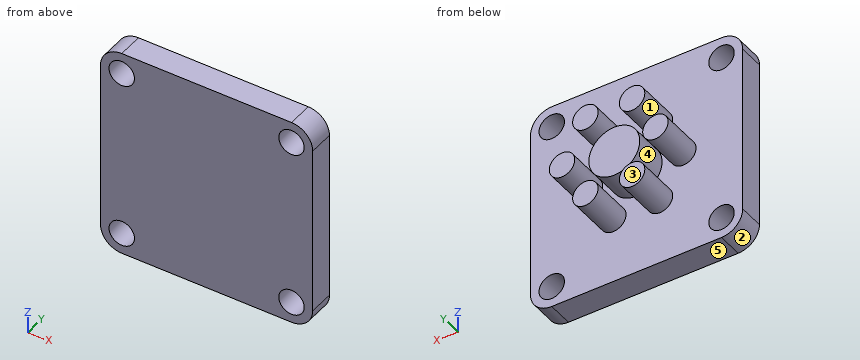
Autodesk Inventor part; units mm, degrees
ref_plane "YZ Plane" through (0, 0, 0) normal (1, 0, 0) x (0, 1, 0)
ref_plane "XZ Plane" through (0, 0, 0) normal (0, 1, 0) x (-1, 0, 0)
ref_plane "XY Plane" through (0, 0, 0) normal (0, 0, 1) x (1, 0, 0)
sketch "Sketch1" plane through (0, 0, 0) normal (0, 1, 0) x (-1, 0, 0)
  line L0 (-12.5, 12.5) -> (12.5, 12.5)
  line L1 (12.5, 12.5) -> (12.5, -12.5)
  line L2 (12.5, -12.5) -> (-12.5, -12.5)
  line L3 (-12.5, -12.5) -> (-12.5, 12.5)
  line L4 (-12.5, 12.5) -> (12.5, -12.5) construction
  line L5 (12.5, 12.5) -> (-12.5, -12.5) construction
  line L6 (-10, 10) -> (10, 10) construction
  line L7 (10, 10) -> (10, -10) construction
  line L8 (10, -10) -> (-10, -10) construction
  line L9 (-10, -10) -> (-10, 10) construction
  line L10 (-10, 10) -> (10, -10) construction
  line L11 (10, 10) -> (-10, -10) construction
  circle A0 centre (10, 10) radius 1.5
  circle A1 centre (10, -10) radius 1.5
  circle A2 centre (-10, -10) radius 1.5
  circle A3 centre (-10, 10) radius 1.5
  point P0 (0, 0)
  dimension "d0" = 25
  dimension "d1" = 25
  dimension "d2" = 3
  dimension "d3" = 3
  dimension "d4" = 3
  dimension "d5" = 3
  dimension "d6" = 20
extrude "Extrusion1" add sketch "Sketch1" along normal blind 3
sketch "Sketch2" plane through (0, 3, 0) normal (0, 1, 0) x (1, 0, 0)
  circle A0 centre (0, 0) radius 3
  circle A1 centre (-5.5, 0) radius 1.5
  circle A2 centre (-2.75, -4.7631) radius 1.5
  circle A3 centre (2.75, -4.7631) radius 1.5
  circle A4 centre (5.5, 0) radius 1.5
  circle A5 centre (2.75, 4.7631) radius 1.5
  circle A6 centre (-2.75, 4.7631) radius 1.5
  dimension "d9" = 6
  dimension "d10" = 3
  dimension "d11" = 5.5
  dimension "d14" = 360
extrude "Extrusion2" add sketch "Sketch2" along normal blind 5 contours A1 | A2 | A3 | A4 | A5 | A6
sketch "Sketch3" plane through (0, 3, 0) normal (0, 1, 0) x (1, 0, 0)
  circle A0 centre (0, 0) radius 3
  dimension "d18" = 6
extrude "Extrusion3" add sketch "Sketch3" along normal blind 4
sketch "Sketch5" plane through (-5.5, 8, 0) normal (0, 1, 0) x (1, 0, 0)
  circle A0 centre (0, 0) radius 2.5
  circle A1 centre (2.75, -4.7631) radius 2.5
  circle A2 centre (8.25, -4.7631) radius 2.5
  circle A3 centre (11, 0) radius 2.5
  circle A4 centre (8.25, 4.7631) radius 2.5
  circle A5 centre (2.75, 4.7631) radius 2.5
  circle A6 centre (5.5, 0) radius 3.5
  circle A7 centre (0, 0) radius 1.4875
  circle A8 centre (2.75, -4.7631) radius 1.4875
  circle A9 centre (8.25, -4.7631) radius 1.4875
  circle A10 centre (11, 0) radius 1.4875
  circle A11 centre (8.25, 4.7631) radius 1.4875
  circle A12 centre (2.75, 4.7631) radius 1.4875
  line L0 (18, 12.5) -> (-7, 12.5)
  line L1 (18, -12.5) -> (-7, -12.5)
  line L2 (-7, -12.5) -> (-7, 12.5)
  line L3 (-7, 12.5) -> (18, 12.5)
  line L4 (18, 12.5) -> (18, -12.5)
  line L5 (18, -12.5) -> (-7, 12.5) construction
  line L6 (-7, -12.5) -> (18, 12.5) construction
  circle A13 centre (-4.5, -10) radius 1.5
  circle A14 centre (-4.5, -10) radius 1.65
  circle A15 centre (-4.5, 10) radius 1.5
  circle A16 centre (-4.5, 10) radius 1.65
  circle A17 centre (15.5, 10) radius 1.5
  circle A18 centre (15.5, 10) radius 1.65
  circle A19 centre (15.5, -10) radius 1.5
  circle A20 centre (15.5, -10) radius 1.65
  point P0 (8.7955, -1.179)
  point P1 (8.1687, -2.2645)
  point P2 (6.1267, -3.4434)
  point P3 (4.8733, -3.4434)
  point P4 (2.8313, -2.2645)
  point P5 (2.2045, -1.179)
  point P6 (2.2045, 1.179)
  point P7 (2.8313, 2.2645)
  point P8 (4.8733, 3.4434)
  point P9 (6.1267, 3.4434)
  point P10 (8.1687, 2.2645)
  point P11 (8.7955, 1.179)
  dimension "d21" = 5
  dimension "d24" = 360
  dimension "d26" = 7
  dimension "d29" = 360
extrude "Extrusion4" add sketch "Sketch5" against normal blind 5 contours L4 L1 L2 L0 | A14 | A16 | A18 | A20
fillet "Fillet1" radius 0.5 12 edges at (-2.6687, 5.5, 2.2645) (-0.6267, 5.5, 3.4434) (2.6687, 5.5, 2.2645) (0.6267, 5.5, 3.4434) (-3.2955, 5.5, -1.179) (-3.2955, 5.5, 1.179) (-0.6267, 5.5, -3.4434) (-2.6687, 5.5, -2.2645) (2.6687, 5.5, -2.2645) (0.6267, 5.5, -3.4434) (3.2955, 5.5, 1.179) (3.2955, 5.5, -1.179)
fillet "Fillet2" radius 2.5 4 edges at (12.5, 4, -12.5) (-12.5, 4, -12.5) (12.5, 4, 12.5) (-12.5, 4, 12.5)
sketch "Sketch7" plane through (0, 7, 0) normal (0, 1, 0) x (1, 0, 0)
  circle A0 centre (0, 0) radius 1
extrude "Extrusion5" [suppressed]
sketch "Sketch8" plane through (-5.5, 8, 0) normal (0, 1, 0) x (1, 0, 0)
  circle A0 centre (0, 0) radius 1
  point P0 (5.5, 0)
  dimension "d37" = 2
extrude "Extrusion6" [suppressed]
pattern_circular "Circular Pattern1" [suppressed]
sketch "Sketch9" plane through (-5.5, 8, 0) normal (0, 1, 0) x (1, 0, 0)
  line L0 (-7.0276, -1) -> (-2, -1)
  line L1 (-2, -1) -> (-2, 1)
  line L2 (-2, 1) -> (-7.0276, 1)
  line L3 (-7.0276, 1) -> (-7.0276, -1)
  line L4 (-7.0276, -1) -> (-2, 1) construction
  line L5 (-2, -1) -> (-7.0276, 1) construction
  point P0 (5.5, 0)
  point P1 (-4.5138, 0)
extrude "Extrusion7" cut sketch "Sketch9" against normal blind 5
thicken "Thicken1" operation add thickness 5 both sides no extend neighbours yes toward (0, -1, 0) faces at (0.7594, 8, 10.7394)
properties part number "PDMS stretcher mould A"
The model under review builds one solid part; all positions refer to its coordinate system, in mm. Face numbers are marked on the shaded views. A direction names the side the tool comes from. Give positions to 0.01 mm unless a question says otherwise; leave off trailing zeros. Write each loop counter-clockwise with the first axis right and the second up, starting at its lowest first coordinate (ties: lowest second). Pieces come first, ordered by that corner, then holes. Notation, with made-up numbers: (-1, 18.25) - (44, 18.25) arc R8 ccw to (44, 27.25) - close; hole circle Ø4 at (59, 88.25). An arc over 180 degrees is marked (long way). Answer in a Markdown table with one row per item. Add a question column.
1. Wall thickness on line 1 along X through (y, z) = (5.75, 0); line 2 along Z through (x, y) = (10, 1.55): over which ranges is each line inside the solid? List them lowest first. Write a range as [from, to].
2. We need section C-C on x = -9. Write out the cut boundary in (y, z).
3. We need section A-A on x = -5.5. Write out the cut boundary in (y, z).
4. Tool access review of the marked faces 4 and 5: name each direction out of +Z, -Z, +X, -X, +Y, -Y from which nothing blocks a thin tool from reaching the whole face with its end or side.
5. Insertion check: P1, Ø1.8, axis at x = 0, z = -1.5, coming from the +Y side; P2, Ø1, axis at x = -0.5, y = 6.5, coming from the -Z side; P3, Ø4, axis at x = -10, z = 10, coming from the +Y side. Each pin has a flat end and moves straight along its axis. Give the tip position at first contact, or say it passes through.
6. We need section B-B on y = 6.25. Write out the cut boundary in (x, z).
7. We need section D-D on z = 0.5. Write out the cut boundary in (x, y), then the cut area to 3 significant figures.
8. Draft analysis for pull direction Z (two halves, no side actions). For the marked faces 1, 2 and 3, state which applies: +Z half, -Z half, draft (parallel to the pull), parting line (faces both ways), or undercut.
Ans:
| question | item | result |
|---|---|---|
| 1 | line 1 | x = [-7, -4], [-3, 3], [4, 7] |
| 1 | line 2 | z = [-12.5, -11.5], [-8.5, 8.5], [11.5, 12.5] |
| 2 | outline | (0, -12.5) - (3, -12.5) - (3, -11.12) - (0, -11.12) - close; (0, -8.88) - (3, -8.88) - (3, 8.88) - (0, 8.88) - close; (0, 11.12) - (3, 11.12) - (3, 12.5) - (0, 12.5) - close |
| 3 | outline | (0, -12.5) - (3, -12.5) - (3, -1.5) - (8, -1.5) - (8, 1.5) - (3, 1.5) - (3, 12.5) - (0, 12.5) - close |
| 4 | face 4 | +Y |
| 4 | face 5 | -Z, +X, -X, +Y, -Y |
| 5 | P1 | stops at y = 7 |
| 5 | P2 | stops at z = -3 |
| 5 | P3 | stops at y = 3 |
| 6 | outline | circle Ø3 at (-5.5, 0); circle Ø3 at (-2.75, -4.76); circle Ø3 at (-2.75, 4.76); circle Ø6 at (0, 0); circle Ø3 at (2.75, -4.76); circle Ø3 at (2.75, 4.76); circle Ø3 at (5.5, 0) |
| 7 | outline | (-12.5, 0) - (12.5, 0) - (12.5, 3) - (6.91, 3) - (6.91, 8) - (4.09, 8) - (4.09, 3) - (2.96, 3) - (2.96, 7) - (-2.96, 7) - (-2.96, 3) - (-4.09, 3) - (-4.09, 8) - (-6.91, 8) - (-6.91, 3) - (-12.5, 3) - close |
| 7 | area | 127 mm^2 |
| 8 | face 1 | undercut |
| 8 | face 2 | -Z half |
| 8 | face 3 | draft |
